```python
from build123d import *

# Parameters (mm, degrees)
SKETCH1_R           = 1.85
BOSS_EXTRUDE1_DEPTH = 3.1
SKETCH2_R           = 1.5
BOSS_EXTRUDE2_DEPTH = 1
SKETCH3_R           = 1.1
BOSS_EXTRUDE3_DEPTH = 2
SKETCH6_W           = 5
SKETCH6_H           = 5
BOSS_EXTRUDE4_DEPTH = 50
SKETCH7_R           = 1
CUT_EXTRUDE1_DEPTH  = 24


with BuildPart() as part:
    # Sketch1 → Boss-Extrude1 (new body)
    with BuildSketch(Plane(origin=(0, 0, 0), x_dir=(1, 0, 0), z_dir=(0, 1, 0))):
        with Locations(Location((0, 0, 0), (0, 0, 90))):
            Circle(SKETCH1_R)
    extrude(amount=BOSS_EXTRUDE1_DEPTH)

    # Sketch2 → Boss-Extrude2 (add)
    with BuildSketch(Plane(origin=(0, 3.1, 0), x_dir=(1, 0, 0), z_dir=(0, 1, 0))):
        with Locations(Location((0, 0, 0), (0, 0, 270))):
            Circle(SKETCH2_R)
    extrude(amount=BOSS_EXTRUDE2_DEPTH)

    # Sketch3 → Boss-Extrude3 (add)
    with BuildSketch(Plane(origin=(0, 4.1, 0), x_dir=(1, 0, 0), z_dir=(0, 1, 0))):
        with Locations(Location((0, 0, 0), (0, 0, 270))):
            Circle(SKETCH3_R)
    extrude(amount=BOSS_EXTRUDE3_DEPTH)

    # Loft1: read off the stored shape, not the designer's step
    # Loft1: loft between two sections, ruled curve by curve
    loft1_from = [
        Edge.make_bspline([(0, 6.1, 1.85), (3.7, 6.1, 1.85), (3.7, 6.1, -1.85), (0, 6.1, -1.85), (-3.7, 6.1, -1.85), (-3.7, 6.1, 1.85), (0, 6.1, 1.85)], [0, 0, 0, 0, 0.5, 0.5, 0.5, 1, 1, 1, 1], 3, [1, 0.333333333, 0.333333333, 1, 0.333333333, 0.333333333, 1]),
    ]
    loft1_to = [
        Edge.make_bspline([(0.620465421, 8.6, 0.968257539), (2.556980499, 8.6, -0.272673303), (1.316049657, 8.6, -2.209188381), (-0.620465421, 8.6, -0.968257539), (-2.556980499, 8.6, 0.272673303), (-1.316049657, 8.6, 2.209188381), (0.620465421, 8.6, 0.968257539)], [0, 0, 0, 0, 0.5, 0.5, 0.5, 1, 1, 1, 1], 3, [1, 0.333333333, 0.333333333, 1, 0.333333333, 0.333333333, 1]),
    ]
    loft1 = Solid(Shell([*[Face.make_surface_from_curves(loft1_from[k], loft1_to[k]) for k in range(1)], Face(Wire(loft1_from)), Face(Wire(loft1_to))]))
    add(loft1)

    # Sketch6 → Boss-Extrude4 (add)
    with BuildSketch(Plane.XZ):
        Rectangle(SKETCH6_W, SKETCH6_H)
    extrude(amount=BOSS_EXTRUDE4_DEPTH)

    # Sketch7 → Cut-Extrude1 (cut)
    with BuildSketch(Plane.XZ.offset(50)):
        with Locations(Location((0, 0, 0), (0, 0, 270))):
            Circle(SKETCH7_R)
    extrude(amount=-CUT_EXTRUDE1_DEPTH, mode=Mode.SUBTRACT)


solid = part.part
```
For this review, take the finished solid that the model builds, in its own axes (mm). A direction names the side the tool comes from. Give positions to 0.01 mm unless a question says otherwise; leave off trailing zeros. Write each loop counter-clockwise with the first axis right and the second up, starting at its lowest first coordinate (ties: lowest second). Pieces come first, ordered by that corner, then holes. Notation, with made-up numbers: M 64,85 L 110,85 A15 ccw 110,102 Z; hole C -34.75,-19.5 d3. An arc over 180 degrees is marked long. Answer as a JSON object with one key per item and string values. Group by question number.
Item 1: For probe 1 along X at (y, z) = (-39, 0); probe 2 along Z at (x, y) = (0.1, 5.5); probe 3 along Y at (x, z) = (-0.1, 0.5), list the stretches that pass through material, from the lowest coordinate up. Write a range as [from, to].
Item 2: Consider section A-A on y = -26.5. Write out the cut boundary in (x, z), plus the area to 3 significant figures.
Item 3: Tool access review of faces 4 (the cylindrical face through (1.806, 1.528, 0.401)), 5 (the flat face through (0, -26, 0)), 6 (the flat face through (1, 6.1, 1)), 7 (the flat face through (0, 8.6, 0)), 8 (the flat face through (2.5, -25, 0)): name each direction out of +Z, -Z, +X, -X, +Y, -Y from which nothing blocks a thin tool from reaching the whole face with its end or side.
Item 4: Draft analysis for pull direction Y (two halves, no side actions). For faces 1 (the cylindrical face through (0.45, 3.59, 1.43)), 2 (the flat face through (1, 0, 2)), 3 (the flat face through (-2.5, -25, 0)), state which applies: +Y half, -Y half, draft (parallel to the pull), parting line (faces both ways), or undercut.
Item 5: For pin 1 Ø0.6 at (x, z) = (0, 0) entering from -Y, flat-tipped, find the tip position at first contact; note if it passes through.
Check result:
{
 "1": {"probe 1": "x = [-2.5, -1], [1, 2.5]", "probe 2": "z = [-1.1, 1.1]", "probe 3": "y = [-26, 8.6]"},
 "2": {"outline": "M -2.5,-2.5 L 2.5,-2.5 L 2.5,2.5 L -2.5,2.5 Z; hole C 0,0 d2", "area": "21.9 mm^2"},
 "3": {"face 4": "+Y", "face 5": "-Y", "face 6": "none", "face 7": "+Z, -Z, +X, -X, +Y", "face 8": "+Z, -Z, +X, +Y, -Y"},
 "4": {"face 1": "undercut", "face 2": "+Y half", "face 3": "draft"},
 "5": {"pin 1": "stops at y = -26"}
}
